from build123d import *

# Parameters (mm, degrees)
BOSS_EXTRUDE1_DEPTH      = 40
BOSS_EXTRUDE1_DEPTH_BACK = 40
SKETCH1_W                = 40
SKETCH1_H                = 5
BOSS_EXTRUDE2_DEPTH      = 2.5
BOSS_EXTRUDE2_DEPTH_BACK = 2.5
SKETCH2_W                = 18
SKETCH2_H                = 25
SKETCH2_R                = 1.75
FILLET1_R                = 1.5
FILLET2_R                = 1.5
FILLET3_R                = 1.5


with BuildPart() as part:
    # Sketch1 → Boss-Extrude1 (new, two sides: drawn at the far end of the back side and taken through both)
    with BuildSketch(Plane.XY.offset(-BOSS_EXTRUDE1_DEPTH_BACK)):
        Rectangle(SKETCH1_W, SKETCH1_H)
    extrude(amount=BOSS_EXTRUDE1_DEPTH + BOSS_EXTRUDE1_DEPTH_BACK)

    # Sketch2 → Boss-Extrude2 (add, two sides: drawn at the far end of the back side and taken through both)
    with BuildSketch(Plane.XY.offset(-BOSS_EXTRUDE2_DEPTH_BACK)):
        with Locations((0, 15)):
            Rectangle(SKETCH2_W, SKETCH2_H)
        with Locations((-5, 11)):
            Circle(SKETCH2_R, mode=Mode.SUBTRACT)
        with Locations((5, 11)):
            Circle(SKETCH2_R, mode=Mode.SUBTRACT)
        with Locations((5, 21)):
            Circle(SKETCH2_R, mode=Mode.SUBTRACT)
        with Locations((-5, 21)):
            Circle(SKETCH2_R, mode=Mode.SUBTRACT)
    extrude(amount=BOSS_EXTRUDE2_DEPTH + BOSS_EXTRUDE2_DEPTH_BACK)

    # Fillet1
    fillet1_edges = [part.edges().sort_by_distance(p)[0] for p in [
        (0, 2.5, 40),
        (0, -2.5, 40),
        (0, -2.5, -40),
        (9, 2.5, 0),
        (0, 2.5, -2.5),
        (-9, 2.5, 0),
        (0, 2.5, 2.5),
        (20, -2.5, 0),
        (-20, -2.5, 0),
        (-20, 2.5, 0),
        (20, 2.5, 0),
        (0, 2.5, -40),
    ]]
    fillet(fillet1_edges, radius=FILLET1_R)

    # Fillet2
    # the kernel refuses this fillet: 1.5 mm, written as the material it takes off along each edge
    with BuildSketch(Plane(origin=(18.5, 1, 38.5), x_dir=(1, 0, 0), z_dir=(0, 0, 1))) as fillet2_piece_1_section:
        Polygon((0, 0), (FILLET2_R, 0), (FILLET2_R, FILLET2_R), (0, FILLET2_R), align=None)
    fillet2_piece_1 = extrude(amount=FILLET2_R, mode=Mode.PRIVATE)
    fillet2_piece_1 = fillet2_piece_1 - Plane(origin=(18.5, 1, 38.5), x_dir=(-0.7071067811865475, -0.7071067811865475, 0), z_dir=(0, 0, 1)) * Sphere(FILLET2_R, mode=Mode.PRIVATE)
    add(fillet2_piece_1, mode=Mode.SUBTRACT)
    with BuildSketch(Plane(origin=(-18.5, 1, 38.5), x_dir=(-1, 0, 0), z_dir=(0, 0, 1))) as fillet2_piece_2_section:
        Polygon((0, 0), (FILLET2_R, 0), (FILLET2_R, -FILLET2_R), (0, -FILLET2_R), align=None)
    fillet2_piece_2 = extrude(amount=FILLET2_R, mode=Mode.PRIVATE)
    fillet2_piece_2 = fillet2_piece_2 - Plane(origin=(-18.5, 1, 38.5), x_dir=(0.7071067811865475, -0.7071067811865475, 0), z_dir=(0, 0, 1)) * Sphere(FILLET2_R, mode=Mode.PRIVATE)
    add(fillet2_piece_2, mode=Mode.SUBTRACT)
    with BuildSketch(Plane(origin=(-18.5, -1, 38.5), x_dir=(-1, 0, 0), z_dir=(0, 0, 1))) as fillet2_piece_3_section:
        Polygon((0, 0), (FILLET2_R, 0), (FILLET2_R, FILLET2_R), (0, FILLET2_R), align=None)
    fillet2_piece_3 = extrude(amount=FILLET2_R, mode=Mode.PRIVATE)
    fillet2_piece_3 = fillet2_piece_3 - Plane(origin=(-18.5, -1, 38.5), x_dir=(0.7071067811865475, 0.7071067811865475, 0), z_dir=(0, 0, 1)) * Sphere(FILLET2_R, mode=Mode.PRIVATE)
    add(fillet2_piece_3, mode=Mode.SUBTRACT)
    with BuildSketch(Plane(origin=(18.5, -1, 38.5), x_dir=(1, 0, 0), z_dir=(0, 0, 1))) as fillet2_piece_4_section:
        Polygon((0, 0), (FILLET2_R, 0), (FILLET2_R, -FILLET2_R), (0, -FILLET2_R), align=None)
    fillet2_piece_4 = extrude(amount=FILLET2_R, mode=Mode.PRIVATE)
    fillet2_piece_4 = fillet2_piece_4 - Plane(origin=(18.5, -1, 38.5), x_dir=(-0.7071067811865475, 0.7071067811865475, 0), z_dir=(0, 0, 1)) * Sphere(FILLET2_R, mode=Mode.PRIVATE)
    add(fillet2_piece_4, mode=Mode.SUBTRACT)
    with BuildSketch(Plane(origin=(20, 1, 40), x_dir=(-1, 0, 0), z_dir=(0, -1, 0)), Plane(origin=(-20, -1, 40), x_dir=(1, 0, 0), z_dir=(0, 1, 0))) as fillet2_piece_5:
        with BuildLine():
            CenterArc((FILLET2_R, FILLET2_R), FILLET2_R, 180, 90)
            Line((0, FILLET2_R), (0, 0))
            Line((0, 0), (FILLET2_R, 0))
        make_face()
    extrude(amount=2, mode=Mode.SUBTRACT)

    # Fillet3
    # the kernel refuses this fillet: 1.5 mm, written as the material it takes off along each edge
    with BuildSketch(Plane(origin=(18.5, 1, -38.5), x_dir=(0, 0, -1), z_dir=(1, 0, 0))) as fillet3_piece_1_section:
        Polygon((0, 0), (FILLET3_R, 0), (FILLET3_R, FILLET3_R), (0, FILLET3_R), align=None)
    fillet3_piece_1 = extrude(amount=FILLET3_R, mode=Mode.PRIVATE)
    fillet3_piece_1 = fillet3_piece_1 - Plane(origin=(18.5, 1, -38.5), x_dir=(0, -0.7071067811865475, 0.7071067811865475), z_dir=(1, 0, 0)) * Sphere(FILLET3_R, mode=Mode.PRIVATE)
    add(fillet3_piece_1, mode=Mode.SUBTRACT)
    with BuildSketch(Plane(origin=(-18.5, 1, -38.5), x_dir=(0, 0, -1), z_dir=(-1, 0, 0))) as fillet3_piece_2_section:
        Polygon((0, 0), (FILLET3_R, 0), (FILLET3_R, -FILLET3_R), (0, -FILLET3_R), align=None)
    fillet3_piece_2 = extrude(amount=FILLET3_R, mode=Mode.PRIVATE)
    fillet3_piece_2 = fillet3_piece_2 - Plane(origin=(-18.5, 1, -38.5), x_dir=(0, -0.7071067811865475, 0.7071067811865475), z_dir=(-1, 0, 0)) * Sphere(FILLET3_R, mode=Mode.PRIVATE)
    add(fillet3_piece_2, mode=Mode.SUBTRACT)
    with BuildSketch(Plane(origin=(-18.5, -1, -38.5), x_dir=(0, 0, -1), z_dir=(-1, 0, 0))) as fillet3_piece_3_section:
        Polygon((0, 0), (FILLET3_R, 0), (FILLET3_R, FILLET3_R), (0, FILLET3_R), align=None)
    fillet3_piece_3 = extrude(amount=FILLET3_R, mode=Mode.PRIVATE)
    fillet3_piece_3 = fillet3_piece_3 - Plane(origin=(-18.5, -1, -38.5), x_dir=(0, 0.7071067811865475, 0.7071067811865475), z_dir=(-1, 0, 0)) * Sphere(FILLET3_R, mode=Mode.PRIVATE)
    add(fillet3_piece_3, mode=Mode.SUBTRACT)
    with BuildSketch(Plane(origin=(18.5, -1, -38.5), x_dir=(0, 0, -1), z_dir=(1, 0, 0))) as fillet3_piece_4_section:
        Polygon((0, 0), (FILLET3_R, 0), (FILLET3_R, -FILLET3_R), (0, -FILLET3_R), align=None)
    fillet3_piece_4 = extrude(amount=FILLET3_R, mode=Mode.PRIVATE)
    fillet3_piece_4 = fillet3_piece_4 - Plane(origin=(18.5, -1, -38.5), x_dir=(0, 0.7071067811865475, 0.7071067811865475), z_dir=(1, 0, 0)) * Sphere(FILLET3_R, mode=Mode.PRIVATE)
    add(fillet3_piece_4, mode=Mode.SUBTRACT)
    with BuildSketch(Plane(origin=(20, 1, -40), x_dir=(0, 0, 1), z_dir=(0, -1, 0)), Plane(origin=(-20, -1, -40), x_dir=(0, 0, 1), z_dir=(0, 1, 0))) as fillet3_piece_5:
        with BuildLine():
            CenterArc((FILLET3_R, FILLET3_R), FILLET3_R, 180, 90)
            Line((0, FILLET3_R), (0, 0))
            Line((0, 0), (FILLET3_R, 0))
        make_face()
    extrude(amount=2, mode=Mode.SUBTRACT)


solid = part.part
The model under review builds one solid part; all positions refer to its coordinate system, in mm. A direction names the side the tool comes from. Give positions to 0.01 mm unless a question says otherwise; leave off trailing zeros. Loops run counter-clockwise (first coordinate to the right, second up) from the corner with the lowest first, then second, coordinate; pieces in that order, holes last. Notation, with made-up numbers: (-12.75, 40.25) -> (12.25, 40.25) arc R4 ccw to (12.25, 45.25) -> close; hole circle Ø5 at (-2.5, 31.5). An arc over 180 degrees is marked (long way). Put each result on its own line as item: value. Start each with the question number.
1. We need section B-B on x = 5. State the section outline as (y, z) points, then the cut area to 3 significant figures.
2. We need section A-A on y = 21. State the section outline as (x, z) points, then the cut area to 3 significant figures.
3. Wall thickness on probe 1 along Y at (x, z) = (5, -0.4); probe 2 along X at (y, z) = (10.25, -2); probe 3 along Y at (x, z) = (-1, 16.5): over which ranges is each line inside the solid? List them lowest first.
4. We need section D-D on x = 17. State the section outline as (y, z) points.
5. For faces 1 (the face through (-20, 0, -1)), 2 (the face through (-9, 16, 0)), list the 3-axis set-ups (+Z, -Z, +X, -X, +Y, -Y) from which the entire face can be reached by the end or side of a thin tool; tool diameter is ignored.
6. Mouldability with a two-part tool opening along Y and no side actions: class faces 3 (the face through (-19.57, -0.01, 39.55)), 4 (the face through (9.653, 2.762, 0.056)), 5 (the face through (-5.228, 22.735, -0.035)), 6 (the face through (3.71, 12.18, -0.04)) as released by +Y, released by -Y, zero draft, split by the parting line, or undercut.
7. Clearance check with flat-ended pins moving along their axes: P1, Ø1, axis at x = 11.5, z = 23.5, coming from the +Y side; P2, Ø2, axis at x = 0.5, y = 2.5, coming from the +Z side; P3, Ø4, axis at y = 10.5, z = -1, coming from the +X side. State where each tip first meets the part, or that it passes through.
8. We need section C-C on z = 32. State the section outline as (x, y) points, then the cut area to 3 significant figures.
Determined:
1. outline: (-2.5, -38.5) arc R1.5 ccw to (-1, -40) -> (1, -40) arc R1.5 ccw to (2.5, -38.5) -> (2.5, -4) arc R1.5 cw to (4, -2.5) -> (9.25, -2.5) -> (9.25, 2.5) -> (4, 2.5) arc R1.5 cw to (2.5, 4) -> (2.5, 38.5) arc R1.5 ccw to (1, 40) -> (-1, 40) arc R1.5 ccw to (-2.5, 38.5) -> close; (12.75, -2.5) -> (19.25, -2.5) -> (19.25, 2.5) -> (12.75, 2.5) -> close; (22.75, -2.5) -> (27.5, -2.5) -> (27.5, 2.5) -> (22.75, 2.5) -> close
1. area: 489 mm^2
2. outline: (-9, -2.5) -> (-6.75, -2.5) -> (-6.75, 2.5) -> (-9, 2.5) -> close; (-3.25, -2.5) -> (3.25, -2.5) -> (3.25, 2.5) -> (-3.25, 2.5) -> close; (6.75, -2.5) -> (9, -2.5) -> (9, 2.5) -> (6.75, 2.5) -> close
2. area: 55.0 mm^2
3. probe 1: -2.5 to 9.25, 12.75 to 19.25, 22.75 to 27.5
3. probe 2: -9 to -6.58, -3.42 to 3.42, 6.58 to 9
3. probe 3: -2.5 to 2.5
4. outline: (-2.5, -38.5) arc R1.5 ccw to (-1, -40) -> (1, -40) arc R1.5 ccw to (2.5, -38.5) -> (2.5, 38.5) arc R1.5 ccw to (1, 40) -> (-1, 40) arc R1.5 ccw to (-2.5, 38.5) -> close
5. face 1: +Z, -Z, -X, +Y, -Y
5. face 2: +Z, -Z, -X, +Y
6. face 3: zero draft
6. face 4: released by +Y
6. face 5: undercut
6. face 6: undercut
7. P1: y = 2.5
7. P2: z = 39.91
7. P3: x = 9
8. outline: (-20, -1) arc R1.5 ccw to (-18.5, -2.5) -> (18.5, -2.5) arc R1.5 ccw to (20, -1) -> (20, 1) arc R1.5 ccw to (18.5, 2.5) -> (-18.5, 2.5) arc R1.5 ccw to (-20, 1) -> close
8. area: 198 mm^2
